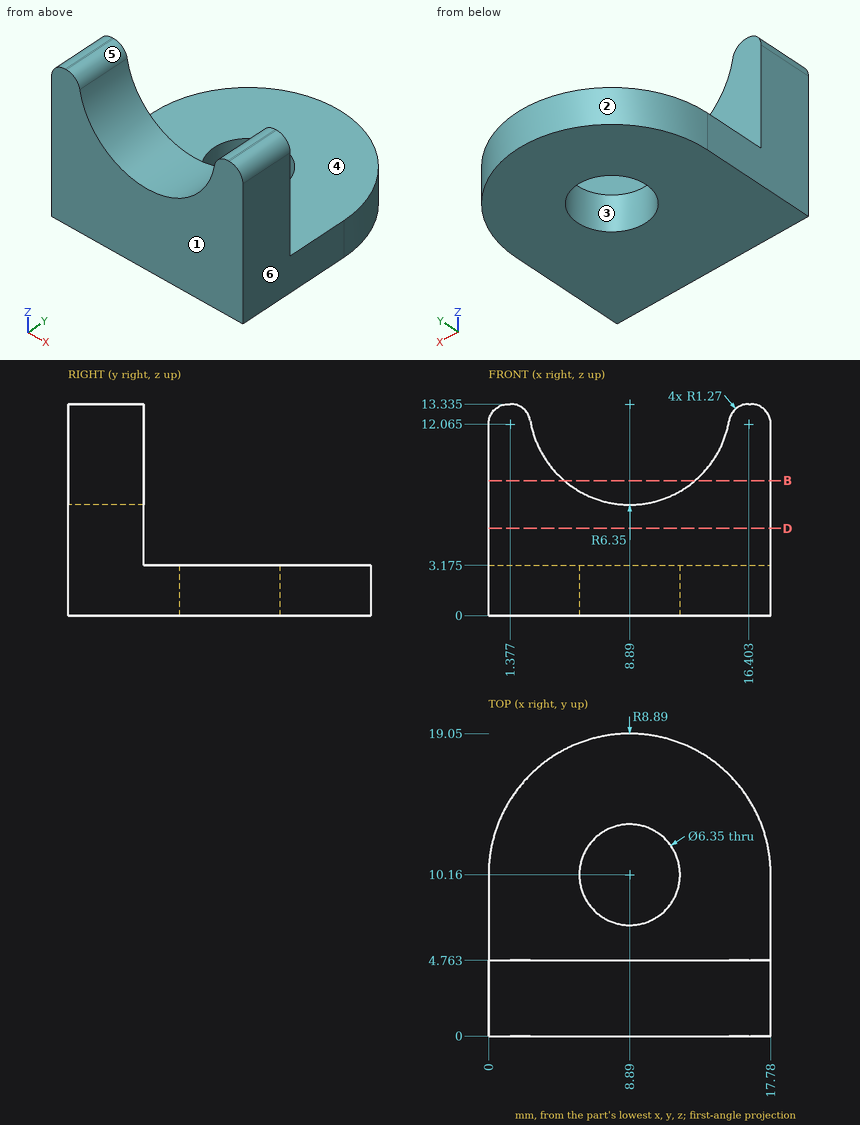
Verification items for this drawing (mm, ordinates from the low corner). A direction names the side the tool comes from. Coordinates: 2 decimals unless noted, no trailing zeros. Order: outer loops, then holes, each group sorted by start corner. A loop starts at its lowest first (then second) coordinate and runs counter-clockwise, first axis right, second up. Notation, with made-up numbers: (48, 87.5) -> (86, 87.5) arc R23 ccw to (86, 116.5) -> close; hole circle Ø2 at (-31.5, 8). An arc over 180 degrees is marked (long way). Put each result on its own line as item: value. Start each with the question number.
1. Mould release check, pull along Y, two halves, no side actions. Record for the marked faces 1, 2 and 3: released by +Y, released by -Y, zero draft, split by the parting line, or undercut.
2. Material ranges on L1, parallel to Y at x = 10, z = 7; L2, parallel to Z at x = 4.5, y = 15.25 (1 decimal); L3, parallel to X at y = 2.5, z = 11.75, recorded low to high. Write a range as [from, to].
3. Cross-section at D-D, the plane z = 5.5. Record the boundary of the cut face in (x, y).
4. Go/stop test with flat-tipped pins: pin 1 Ø3 at (x, z) = (13.5, 5) entering from +Y; pin 2 Ø5 at (x, y) = (14, 12) entering from +Z (1 decimal); pin 3 Ø1 at (x, y) = (2.5, 11) entering from -Z. Record where each tip stops, or that it passes through.
5. Cross-section at B-B, the plane z = 8.5. Record the boundary of the cut face in (x, y).
6. Access from +Z, -Z, +X, -X, +Y, -Y to the whole of each face (thin tool, end or side, straight path). Record for the marked faces 4, 5 and 6.
Computed:
1. face 1: released by -Y
1. face 2: released by +Y
1. face 3: undercut
2. L1: [0, 4.76]
2. L2: [0, 3.2]
2. L3: [0, 2.74], [15.04, 17.78]
3. outline: (0, 0) -> (17.78, 0) -> (17.78, 4.76) -> (0, 4.76) -> close
4. pin 1: y = 4.76
4. pin 2: z = 3.2
4. pin 3: z = 0
5. outline: (0, 0) -> (4.77, 0) -> (4.77, 4.76) -> (0, 4.76) -> close; (13.01, 0) -> (17.78, 0) -> (17.78, 4.76) -> (13.01, 4.76) -> close
6. face 4: +Z, +X, -X, +Y
6. face 5: +Z, +Y, -Y
6. face 6: +Z, -Z, +X, +Y, -Y
